from build123d import *

# Parameters (mm, degrees)
BOSS_EXTRUDE1_DEPTH = 12
CUT_EXTRUDE1_DEPTH  = 13


with BuildPart() as part:
    # Sketch1 → Boss-Extrude1 (new body)
    with BuildSketch(Plane(origin=(0, 0, 0), x_dir=(1, 0, 0), z_dir=(0, 1, 0))):
        with BuildLine():
            Line((-0.551192068, 17.450239661), (-0.551192068, 11.450239661))
            ThreePointArc((-0.551192068, 11.450239661), (-2.978402467, 11.069820222), (-5.268807469, 10.180936541))
            Line((-5.268807469, 10.180936541), (-8.268250593, 15.376124426))
            ThreePointArc((-8.268250593, 15.376124426), (-9.370925272, 16.20727377), (-9.202466164, 14.836754815))
            Line((-9.202466164, 14.836754815), (-6.202466164, 9.640602392))
            ThreePointArc((-6.202466164, 9.640602392), (-8.11428231, 8.097544294), (-9.653389387, 6.182545944))
            Line((-9.653389387, 6.182545944), (-14.848577272, 9.181989068))
            ThreePointArc((-14.848577272, 9.181989068), (-16.219096227, 9.350448175), (-15.387946883, 8.247773497))
            Line((-15.387946883, 8.247773497), (-10.19179446, 5.247773497))
            ThreePointArc((-10.19179446, 5.247773497), (-11.075946761, 2.955537911), (-11.451353414, 0.527547154))
            Line((-11.451353414, 0.527547154), (-17.450239661, 0.527547154))
            ThreePointArc((-17.450239661, 0.527547154), (-18.721373447, -0.011822457), (-17.450239661, -0.551192068))
            Line((-17.450239661, -0.551192068), (-11.450239661, -0.551192068))
            ThreePointArc((-11.450239661, -0.551192068), (-11.069820222, -2.978402467), (-10.180936541, -5.268807469))
            Line((-10.180936541, -5.268807469), (-15.376124426, -8.268250593))
            ThreePointArc((-15.376124426, -8.268250593), (-16.20727377, -9.370925272), (-14.836754815, -9.202466164))
            Line((-14.836754815, -9.202466164), (-9.640602392, -6.202466164))
            ThreePointArc((-9.640602392, -6.202466164), (-8.097544294, -8.11428231), (-6.182545944, -9.653389387))
            Line((-6.182545944, -9.653389387), (-9.181989068, -14.848577272))
            ThreePointArc((-9.181989068, -14.848577272), (-9.350448175, -16.219096227), (-8.247773497, -15.387946883))
            Line((-8.247773497, -15.387946883), (-5.247773497, -10.19179446))
            ThreePointArc((-5.247773497, -10.19179446), (-2.955537911, -11.075946761), (-0.527547154, -11.451353414))
            Line((-0.527547154, -11.451353414), (-0.527547154, -17.450239661))
            ThreePointArc((-0.527547154, -17.450239661), (0.011822457, -18.721373447), (0.551192068, -17.450239661))
            Line((0.551192068, -17.450239661), (0.551192068, -11.450239661))
            ThreePointArc((0.551192068, -11.450239661), (2.978402467, -11.069820222), (5.268807469, -10.180936541))
            Line((5.268807469, -10.180936541), (8.268250593, -15.376124426))
            ThreePointArc((8.268250593, -15.376124426), (9.370925272, -16.20727377), (9.202466164, -14.836754815))
            Line((9.202466164, -14.836754815), (6.202466164, -9.640602392))
            ThreePointArc((6.202466164, -9.640602392), (8.11428231, -8.097544294), (9.653389387, -6.182545944))
            Line((9.653389387, -6.182545944), (14.848577272, -9.181989068))
            ThreePointArc((14.848577272, -9.181989068), (16.219096227, -9.350448175), (15.387946883, -8.247773497))
            Line((15.387946883, -8.247773497), (10.19179446, -5.247773497))
            ThreePointArc((10.19179446, -5.247773497), (11.075946761, -2.955537911), (11.451353414, -0.527547154))
            Line((11.451353414, -0.527547154), (17.450239661, -0.527547154))
            ThreePointArc((17.450239661, -0.527547154), (18.721373447, 0.011822457), (17.450239661, 0.551192068))
            Line((17.450239661, 0.551192068), (11.450239661, 0.551192068))
            ThreePointArc((11.450239661, 0.551192068), (11.069820222, 2.978402467), (10.180936541, 5.268807469))
            Line((10.180936541, 5.268807469), (15.376124426, 8.268250593))
            ThreePointArc((15.376124426, 8.268250593), (16.20727377, 9.370925272), (14.836754815, 9.202466164))
            Line((14.836754815, 9.202466164), (9.640602392, 6.202466164))
            ThreePointArc((9.640602392, 6.202466164), (8.097544294, 8.11428231), (6.182545944, 9.653389387))
            Line((6.182545944, 9.653389387), (9.181989068, 14.848577272))
            ThreePointArc((9.181989068, 14.848577272), (9.350448175, 16.219096227), (8.247773497, 15.387946883))
            Line((8.247773497, 15.387946883), (5.247773497, 10.19179446))
            ThreePointArc((5.247773497, 10.19179446), (2.955537911, 11.075946761), (0.527547154, 11.451353414))
            Line((0.527547154, 11.451353414), (0.527547154, 17.450239661))
            ThreePointArc((0.527547154, 17.450239661), (-0.011822457, 18.721373447), (-0.551192068, 17.450239661))
        make_face()
    extrude(amount=BOSS_EXTRUDE1_DEPTH)

    # Sketch2 → Cut-Extrude1 (cut, through all)
    with BuildSketch(Plane(origin=(0, 12, 0), x_dir=(1, 0, 0), z_dir=(0, 1, 0))):
        with BuildLine():
            Line((-2.236067977, 2), (2.236067977, 2))
            ThreePointArc((2.236067977, 2), (0, -3), (-2.236067977, 2))
        make_face()
    extrude(amount=-CUT_EXTRUDE1_DEPTH, mode=Mode.SUBTRACT)


solid = part.part
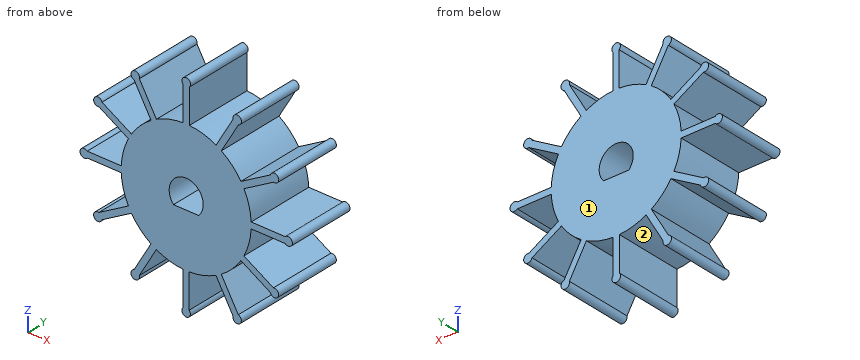
Can you work these out from the model? Positions are in its coordinate system, mm. Face numbers are marked on the shaded views. Coordinates: 2 decimals unless noted, no trailing zeros. Write each loop counter-clockwise with the first axis right and the second up, starting at its lowest first coordinate (ties: lowest second). Pieces come first, ordered by that corner, then holes. Notation, with made-up numbers: (42, 33.5) -> (47, 33.5) arc R15 cw to (47, 55.5) -> close; hole circle Ø2 at (78, -3). An arc over 180 degrees is marked (long way). Write each question's results on one line, items separated by ' | '. Start each with the question number.
Item 1: If we section it at A-A, the plane z = 7: Write out the boundary of the cut face in (x, y), and give its area (3 significant figures).
Item 2: Please list where these lines run through material, in increasing order: probe 1 along Z at (x, y) = (-15.5, 10); probe 2 along X at (y, z) = (3.75, 0); probe 3 along Z at (x, y) = (0, 2.5).
Item 3: I'm going to push flat-ended pins straight in: P1, Ø6.5, axis at y = 3.5, z = 14, coming from the +X side; P2, Ø1, axis at y = 3.5, z = 11, coming from the +X side; P3, Ø8, axis at x = -12, z = -6, coming from the -Y side; P4, Ø3, axis at y = 9, z = -13.5, coming from the +X side. Where does each tip first touch, or does it pass through?
Item 4: If we section it at B-B, the plane z = 0: Write out the boundary of the cut face in (x, y), and give its area (3 significant figures).
Item 5: If we section it at C-C, the plane x = 0: Write out the boundary of the cut face in (y, z), and give its area (3 significant figures).
Item 6: If we section it at D-D, the plane z = -7.5: Write out the boundary of the cut face in (x, y).
Item 7: Thinking about a two-plate mould opening in X: for the marked faces 1 and 2, which applies, released by +X, released by -X, zero draft, split by the parting line, or undercut?
Answer block:
1) outline: (-13.18, 0) -> (-11.02, 0) -> (-11.02, 12) -> (-13.18, 12) -> close; (-9.08, 0) -> (9.08, 0) -> (9.08, 12) -> (-9.08, 12) -> close; (11.07, 0) -> (13.23, 0) -> (13.23, 12) -> (11.07, 12) -> close | area: 270 mm²
2) probe 1: -9.72 to -8.23, -0.53 to 0.55, 8.25 to 9.74 | probe 2: -18.72 to -3, 3 to 18.72 | probe 3: -18.72 to -2, 3 to 18.72
3) P1: x = 9.75 | P2: x = 7.28 | P3: y = 0 | P4: x = 9.46
4) outline: (-18.72, 0) -> (-3, 0) -> (-3, 12) -> (-18.72, 12) -> close; (3, 0) -> (18.72, 0) -> (18.72, 12) -> (3, 12) -> close | area: 377 mm²
5) outline: (0, -18.72) -> (12, -18.72) -> (12, -2) -> (0, -2) -> close; (0, 3) -> (12, 3) -> (12, 18.72) -> (0, 18.72) -> close | area: 389 mm²
6) outline: (-14.09, 0) -> (-11.94, 0) -> (-11.94, 12) -> (-14.09, 12) -> close; (-8.67, 0) -> (8.67, 0) -> (8.67, 12) -> (-8.67, 12) -> close; (11.89, 0) -> (14.05, 0) -> (14.05, 12) -> (11.89, 12) -> close
7) face 1: zero draft | face 2: undercut
